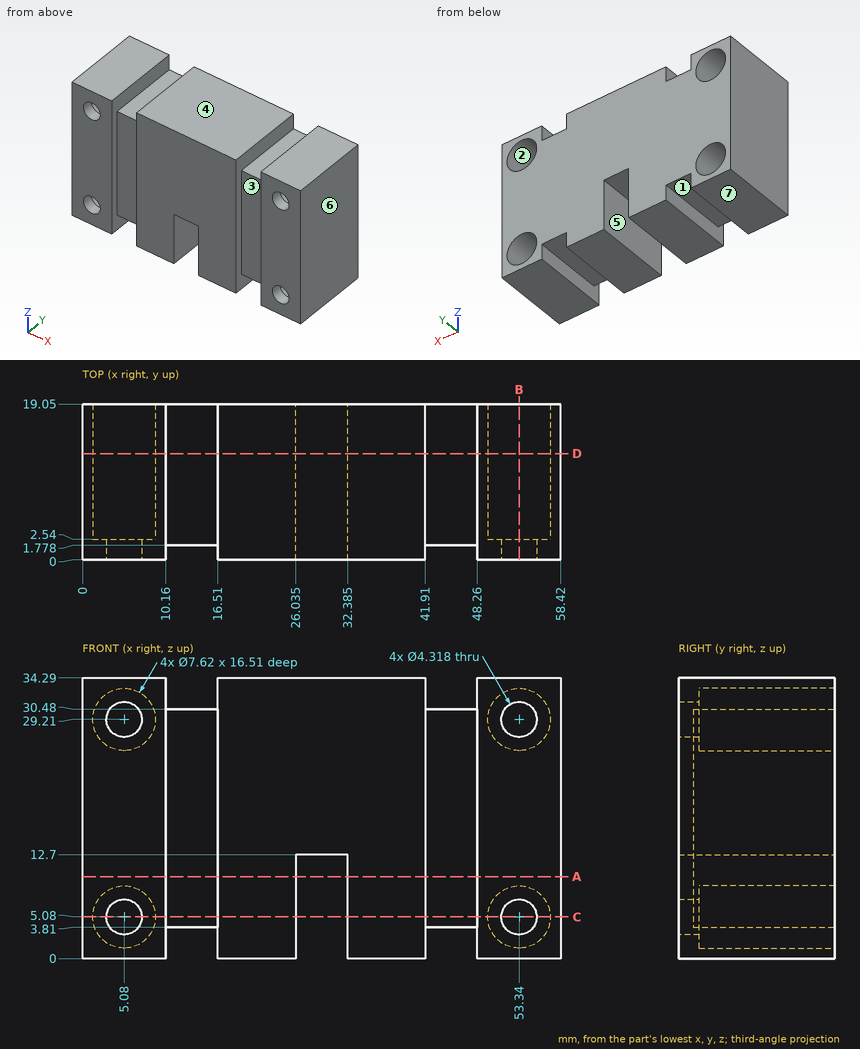
Could you check a few things on this drawing? It's one solid part, dimensions in mm from its lowest x, y, z. A direction names the side the tool comes from. Coordinates: 2 decimals unless noted, no trailing zeros. Order: outer loops, then holes, each group sorted by start corner. A loop starts at its lowest first (then second) coordinate and runs counter-clockwise, first axis right, second up.
1) Imagine slicing it at C-C on z = 5.08. State how many separate pieces and enclosed holes the cut face has, and give its area (3 significant figures).
2) We'd pull the mould along X, two halves only. Please class the marked faces 5, 6 and 7: +X half, -X half, draft (parallel to the pull), parting line (faces both ways), or undercut.
3) I need wall thicknesses on line 1 (Z direction, x = 53.34, y = 0.85); line 2 (X direction, y = 1.6, z = 5.08) (3 decimals); line 3 (X direction, y = 1.5, z = 29.21). Which ranges of each line are inside material? Lowest first, please.
4) Imagine slicing it at A-A on z = 10. List the corners of the cut face in (x, y) for me (3 decimals), and give its area (3 significant figures).
5) Imagine slicing it at D-D on y = 13. List the corners of the cut face in (x, z) for me (3 decimals).
6) Will these pins go through, and if not, where does the flat tip stop? pin 1 (2.5 mm diameter, centred on x = 5.5, z = 6.5, fed in from +Y); pin 2 (3 mm diameter, centred on x = 46, z = 27.5, fed in from -Y); pin 3 (3 mm diameter, centred on x = 46.5, y = 7.5, fed in from -Z).
7) Which directions (+Z, -Z, +X, -X, +Y, -Y) give clear straight access to the entire face, cutting with the end or side of a thin tool? Please do the marked faces 1, 2, 3 and 4.
8) Imagine slicing it at B-B on x = 53.34. List the corners of the cut face in (y, z) for me.
Response values:
1. separate pieces: 4
1. enclosed holes: 0
1. area: 696 mm2
2. face 5: undercut
2. face 6: +X half
2. face 7: draft
3. line 1: z = 0 to 2.92, 7.24 to 27.05, 31.37 to 34.29
3. line 2: x = 0 to 2.921, 7.239 to 10.16, 16.51 to 26.035, 32.385 to 41.91, 48.26 to 51.181, 55.499 to 58.42
3. line 3: x = 0 to 2.92, 7.24 to 10.16, 16.51 to 41.91, 48.26 to 51.18, 55.5 to 58.42
4. outline: (0, 0) - (10.16, 0) - (10.16, 1.778) - (16.51, 1.778) - (16.51, 0) - (26.035, 0) - (26.035, 19.05) - (0, 19.05) - close; (32.385, 0) - (41.91, 0) - (41.91, 1.778) - (48.26, 1.778) - (48.26, 0) - (58.42, 0) - (58.42, 19.05) - (32.385, 19.05) - close
4. area: 969 mm2
5. outline: (0, 0) - (10.16, 0) - (10.16, 3.81) - (16.51, 3.81) - (16.51, 0) - (26.035, 0) - (26.035, 12.7) - (32.385, 12.7) - (32.385, 0) - (41.91, 0) - (41.91, 3.81) - (48.26, 3.81) - (48.26, 0) - (58.42, 0) - (58.42, 34.29) - (48.26, 34.29) - (48.26, 30.48) - (41.91, 30.48) - (41.91, 34.29) - (16.51, 34.29) - (16.51, 30.48) - (10.16, 30.48) - (10.16, 34.29) - (0, 34.29) - close; hole circle Ø7.62 at (5.08, 5.08); hole circle Ø7.62 at (5.08, 29.21); hole circle Ø7.62 at (53.34, 5.08); hole circle Ø7.62 at (53.34, 29.21)
6. pin 1: stops at y = 2.54
6. pin 2: stops at y = 1.78
6. pin 3: stops at z = 3.81
7. face 1: -Z, +Y, -Y
7. face 2: +Y
7. face 3: +Z, -Z, -Y
7. face 4: +Z, +X, -X, +Y, -Y
8. outline: (0, 0) - (19.05, 0) - (19.05, 1.27) - (2.54, 1.27) - (2.54, 2.92) - (0, 2.92) - close; (0, 7.24) - (2.54, 7.24) - (2.54, 8.89) - (19.05, 8.89) - (19.05, 25.4) - (2.54, 25.4) - (2.54, 27.05) - (0, 27.05) - close; (0, 31.37) - (2.54, 31.37) - (2.54, 33.02) - (19.05, 33.02) - (19.05, 34.29) - (0, 34.29) - close
